Answer from the drawing. Dimensions are ordinates in mm from the lowest x, y and z of the part. A direction names the side the tool comes from. Coordinates: 2 decimals unless noted, no trailing zeros. Write each loop counter-clockwise with the first axis right and the second up, starting at its lowest first coordinate (ties: lowest second). Pieces come first, ordered by that corner, then holes. Notation, with made-up numbers: (73, -23) -> (128, -23) arc R36 cw to (128, 16) -> close; hole circle Ø10 at (-33.75, 31). An arc over 180 degrees is marked (long way). One line per item, written item: value. Start each with the question number.
1. For the marked faces 1, 2 and 3, determine the directions among +Z, -Z, +X, -X, +Y, -Y from which every point of the face is accessible in a straight line to the end or side of a thin tool.
2. Find section A-A, the plane y = 3.95. Write down the section's boundary in (x, z).
3. Consider line 1 along X through (y, z) = (2, 15.5); line 2 along Z through (x, y) = (6.75, 1); line 3 along Z through (x, y) = (13, 3). Determine where each line is inside the solid, lowest interval first.
4. Given P1, Ø3.5, axis at x = 15, y = 2.5, coming from the -Z side; P2, Ø8, axis at x = 7.5, z = 6, coming from the -Y side; P3, Ø1.5, axis at y = 3.5, z = 3, coming from the +X side, each flat-ended and moving along its own axis, determine where each tip first touches the part or whether it passes through.
5. Find section B-B, the plane x = 8.25. Write down the section's boundary in (y, z), and give its area (3 significant figures).
6. Find section D-D, the plane x = 10.5. Write down the section's boundary in (y, z).
7. Find section C-C, the plane z = 20. Write down the section's boundary in (x, y), and give its area (3 significant figures).
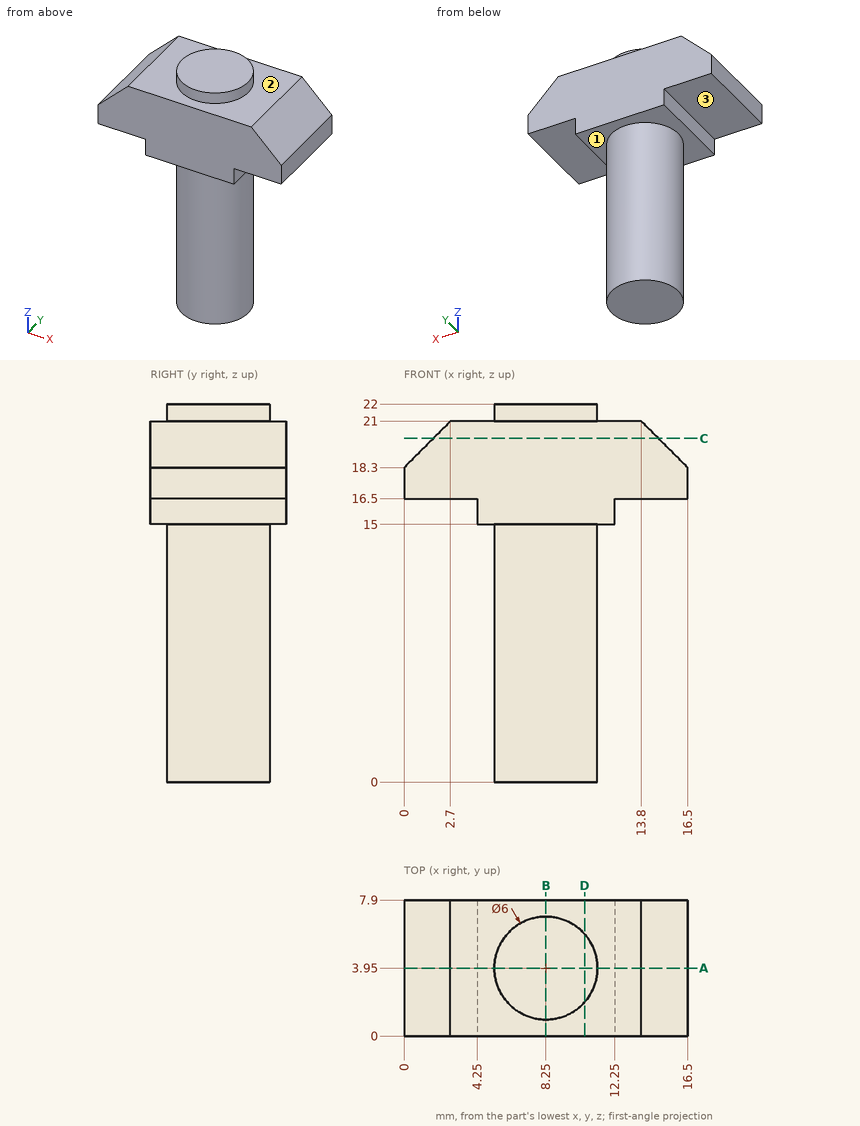
Answer block:
1. face 1: -Z
1. face 2: +Z
1. face 3: -Z, -X, +Y, -Y
2. outline: (0, 16.5) -> (4.25, 16.5) -> (4.25, 15) -> (5.25, 15) -> (5.25, 0) -> (11.25, 0) -> (11.25, 15) -> (12.25, 15) -> (12.25, 16.5) -> (16.5, 16.5) -> (16.5, 18.3) -> (13.8, 21) -> (11.25, 21) -> (11.25, 22) -> (5.25, 22) -> (5.25, 21) -> (2.7, 21) -> (0, 18.3) -> close
3. line 1: x = 4.25 to 12.25
3. line 2: z = 15 to 21
3. line 3: z = 16.5 to 21
4. P1: stops at z = 16.5
4. P2: stops at y = 0.95
4. P3: stops at x = 11.25
5. outline: (0, 15) -> (0.95, 15) -> (0.95, 0) -> (6.95, 0) -> (6.95, 15) -> (7.9, 15) -> (7.9, 21) -> (6.95, 21) -> (6.95, 22) -> (0.95, 22) -> (0.95, 21) -> (0, 21) -> close
5. area: 143 mm2
6. outline: (0, 15) -> (1.97, 15) -> (1.97, 0) -> (5.93, 0) -> (5.93, 15) -> (7.9, 15) -> (7.9, 21) -> (5.93, 21) -> (5.93, 22) -> (1.97, 22) -> (1.97, 21) -> (0, 21) -> close
7. outline: (1.7, 0) -> (14.8, 0) -> (14.8, 7.9) -> (1.7, 7.9) -> close
7. area: 103 mm2
